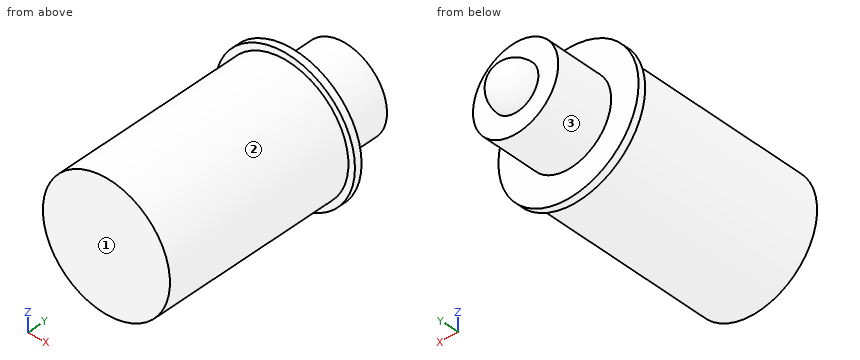
from build123d import *

# Parameters (mm, degrees)
SKETCH1_R           = 2.235
BOSS_EXTRUDE1_DEPTH = 6.75
SKETCH2_R           = 2.465
BOSS_EXTRUDE2_DEPTH = 0.25
SKETCH4_R           = 1.5
BOSS_EXTRUDE3_DEPTH = 2
SKETCH5_R           = 0.8
BOSS_EXTRUDE4_DEPTH = 0.8
FILLET1_R           = 0.8


with BuildPart() as part:
    # Sketch1 → Boss-Extrude1 (new body)
    with BuildSketch(Plane(origin=(0, 0, 0), x_dir=(1, 0, 0), z_dir=(0, 1, 0))):
        with Locations(Location((0, 0, 0), (0, 0, 270))):
            Circle(SKETCH1_R)
    extrude(amount=BOSS_EXTRUDE1_DEPTH)

    # Sketch2 → Boss-Extrude2 (add)
    with BuildSketch(Plane(origin=(0, 6.75, 0), x_dir=(1, 0, 0), z_dir=(0, 1, 0))):
        with Locations(Location((0, 0, 0), (0, 0, 270))):
            Circle(SKETCH2_R)
    extrude(amount=BOSS_EXTRUDE2_DEPTH)

    # Sketch4 → Boss-Extrude3 (add)
    with BuildSketch(Plane(origin=(0, 7, 0), x_dir=(1, 0, 0), z_dir=(0, 1, 0))):
        with Locations(Location((0, 0, 0), (0, 0, 270))):
            Circle(SKETCH4_R)
    extrude(amount=BOSS_EXTRUDE3_DEPTH)

    # Sketch5 → Boss-Extrude4 (add)
    with BuildSketch(Plane(origin=(0, 9, 0), x_dir=(1, 0, 0), z_dir=(0, 1, 0))):
        with Locations(Location((0, 0, 0), (0, 0, 270))):
            Circle(SKETCH5_R)
    extrude(amount=BOSS_EXTRUDE4_DEPTH)

    # Fillet1
    fillet1_edges = [part.edges().sort_by_distance(p)[0] for p in [
        (0, 9.8, -0.8),
    ]]
    fillet(fillet1_edges, radius=FILLET1_R - 0.0001)  # a hair under: the kernel refuses the full size


solid = part.part
Could you check a few things on this model? Use its own coordinates, in mm. Face numbers are marked on the shaded views. A direction names the side the tool comes from. Give positions to 0.01 mm unless a question says otherwise; leave off trailing zeros. Order: outer loops, then holes, each group sorted by start corner. A loop starts at its lowest first (then second) coordinate and runs counter-clockwise, first axis right, second up. Notation, with made-up numbers: (14, -6.5) - (43, -6.5) arc R22 ccw to (43, 18.5) - close; hole circle Ø9 at (-29.5, 68.25). An arc over 180 degrees is marked (long way). Return JSON: item names as keys, results as strings. Group by question number.
Q1. Suppose I cut it at B-B, the plane y = 7.5. Please give me the cut outline in (x, z), and give its area (3 significant figures).
Q2. Suppose I cut it at A-A, the plane z = -1.1. Please give me the cut outline in (x, y), and give its area (3 significant figures).
Q3. Which directions (+Z, -Z, +X, -X, +Y, -Y) give clear straight access to the entire face, cutting with the end or side of a thin tool? Please do the marked faces 1, 2 and 3.
Q4. Will these pins go through, and if not, where does the flat tip stop? pin 1 Ø1 at (x, z) = (0, 0) entering from -Y; pin 2 Ø2 at (x, z) = (-1.5, 1.5) entering from +Y; pin 3 Ø1 at (y, z) = (5.5, 0) entering from +X (3 decimals).
Q5. Suppose I cut it at D-D, the plane x = -1.6. Please give me the cut outline in (y, z), and give its area (3 significant figures).
Q6. Please list where these lines run through material, in increasing order: line 1 along Y through (x, z) = (-1.95, -0.6); line 2 along Y through (x, z) = (-1.35, 0.55); line 3 along Z through (x, y) = (0.05, 8). Write a range as [from, to].
Q7. Suppose I cut it at C-C, the plane x = -1.1. Please give me the cut outline in (y, z), and give its area (3 significant figures).
Resolved:
{
 "1": {"outline": "circle Ø3 at (0, 0)", "area": "7.07 mm2"},
 "2": {"outline": "(-2.21, 6.75) - (-1.95, 6.75) - (-1.95, 0) - (1.95, 0) - (1.95, 6.75) - (2.21, 6.75) - (2.21, 7) - (1.02, 7) - (1.02, 9) - (-1.02, 9) - (-1.02, 7) - (-2.21, 7) - close", "area": "31.4 mm2"},
 "3": {"face 1": "+Z, -Z, +X, -X, -Y", "face 2": "-Y", "face 3": "+Y"},
 "4": {"pin 1": "stops at y = 0", "pin 2": "stops at y = 9", "pin 3": "stops at x = 2.235"},
 "5": {"outline": "(0, -1.56) - (6.75, -1.56) - (6.75, -1.88) - (7, -1.88) - (7, 1.88) - (6.75, 1.88) - (6.75, 1.56) - (0, 1.56) - close", "area": "22.0 mm2"},
 "6": {"line 1": "y = [0, 7]", "line 2": "y = [0, 9]", "line 3": "z = [-1.5, 1.5]"},
 "7": {"outline": "(0, -1.95) - (6.75, -1.95) - (6.75, -2.21) - (7, -2.21) - (7, -1.02) - (9, -1.02) - (9, 1.02) - (7, 1.02) - (7, 2.21) - (6.75, 2.21) - (6.75, 1.95) - (0, 1.95) - close", "area": "31.4 mm2"}
}
